Can you work these out from the model? Positions are in its coordinate system, mm. A direction names the side the tool comes from. Round coordinates to 2 decimals unless told otherwise and drop trailing zeros. Order: outer loops, then holes, each group sorted by start corner. A loop starts at its lowest first (then second) coordinate and runs counter-clockwise, first axis right, second up. Notation, with made-up numbers: (27.25, 24.5) -> (46.25, 24.5) arc R23 ccw to (46.25, 49.5) -> close; hole circle Ø2 at (-11.75, 75.5). An arc over 180 degrees is marked (long way). One line per item, written item: value.
```python
from build123d import *

# Parameters (mm, degrees)
ESQUISSE1_W      = 60
ESQUISSE1_H      = 33
ESQUISSE1_R      = 1.5
EXTRUSION1_DEPTH = 3
ESQUISSE2_W      = 7.634201779
ESQUISSE2_H      = 7.63420178
ESQUISSE2_W_2    = 5.337752956
ESQUISSE2_H_2    = 14.027301674
ESQUISSE2_W_3    = 5.224355128
ESQUISSE2_H_3    = 5.224355128
EXTRUSION2_DEPTH = 18
ESQUISSE3_R      = 3.279080348
EXTRUSION3_DEPTH = 12
ESQUISSE4_W      = 4
ESQUISSE4_H      = 19.646099489
EXTRUSION4_DEPTH = 23


with BuildPart() as part:
    # Esquisse1 → Extrusion1 (new body)
    with BuildSketch(Plane(origin=(0, 0, 0), x_dir=(1, 0, 0), z_dir=(0, 1, 0))):
        with Locations((30, 16.5)):
            Rectangle(ESQUISSE1_W, ESQUISSE1_H)
        with Locations((2.75, 29.5)):
            Circle(ESQUISSE1_R, mode=Mode.SUBTRACT)
        with Locations((57.25, 29.5)):
            Circle(ESQUISSE1_R, mode=Mode.SUBTRACT)
        with Locations((57.25, 3.5)):
            Circle(ESQUISSE1_R, mode=Mode.SUBTRACT)
        with Locations((2.75, 3.5)):
            Circle(ESQUISSE1_R, mode=Mode.SUBTRACT)
    extrude(amount=EXTRUSION1_DEPTH)

    # Esquisse2 → Extrusion2 (add)
    with BuildSketch(Plane(origin=(0, 3, 0), x_dir=(1, 0, 0), z_dir=(0, 1, 0))):
        with Locations((33.593446124, 26.205676479)):
            Rectangle(ESQUISSE2_W, ESQUISSE2_H)
        with Locations((51.457386868, 17.801055276)):
            Rectangle(ESQUISSE2_W_2, ESQUISSE2_H_2)
        with Locations((11.46939236, 25.577155504)):
            Rectangle(ESQUISSE2_W_3, ESQUISSE2_H_3)
        with Locations((22.552159567, 25.577155504)):
            Rectangle(ESQUISSE2_W_3, ESQUISSE2_H_3)
    extrude(amount=EXTRUSION2_DEPTH)

    # Esquisse3 → Extrusion3 (add)
    with BuildSketch(Plane(origin=(0, 3, 0), x_dir=(1, 0, 0), z_dir=(0, 1, 0))):
        with Locations((14, 8.756763264)):
            Circle(ESQUISSE3_R)
        with Locations((22, 8.756763264)):
            Circle(ESQUISSE3_R)
        with Locations((30, 8.756763264)):
            Circle(ESQUISSE3_R)
        with Locations((38, 8.756763264)):
            Circle(ESQUISSE3_R)
    extrude(amount=EXTRUSION3_DEPTH)

    # Esquisse4 → Extrusion4 (add)
    with BuildSketch(Plane(origin=(0, 3, 0), x_dir=(1, 0, 0), z_dir=(0, 1, 0))):
        with Locations((43.737455539, 15.895279312)):
            Rectangle(ESQUISSE4_W, ESQUISSE4_H)
    extrude(amount=EXTRUSION4_DEPTH)


solid = part.part
```
Q1. I want a section at B-B on z = -3.5. List the corners of the cut face in (x, y) for me, plus the area to 3 significant figures.
Answers below:
outline: (0, 0) -> (1.25, 0) -> (1.25, 3) -> (0, 3) -> close; (4.25, 0) -> (55.75, 0) -> (55.75, 3) -> (4.25, 3) -> close; (58.75, 0) -> (60, 0) -> (60, 3) -> (58.75, 3) -> close
area: 162 mm^2
Q2. I want a section at A-A on x = 2.75. List the corners of the cut face in (y, z) for me, plus the area to 3 significant figures.
Answers below:
outline: (0, -33) -> (3, -33) -> (3, -31) -> (0, -31) -> close; (0, -28) -> (3, -28) -> (3, -5) -> (0, -5) -> close; (0, -2) -> (3, -2) -> (3, 0) -> (0, 0) -> close
area: 81.0 mm^2
Q3. Please list where these lines run through material, in increasing order: line 1 along X through (y, z) = (12, -24.5); line 2 along Z through (x, y) = (57.25, 1.45); line 3 along X through (y, z) = (2.25, -29.5).
Answers below:
line 1: 8.86 to 14.08, 19.94 to 25.16, 29.78 to 37.41, 41.74 to 45.74, 48.79 to 54.13
line 2: -33 to -31, -28 to -5, -2 to 0
line 3: 0 to 1.25, 4.25 to 55.75, 58.75 to 60
Q4. We'd pull the mould along X, two halves only. Please class faces 1 (the face through (8.857, 12, -26)), 2 (the face through (51, 21, -18)), 3 (the face through (58.68, 1.48, -29.95)): released by +X, released by -X, zero draft, split by the parting line, or undercut.
Answers below:
face 1: released by -X
face 2: zero draft
face 3: undercut
Q5. I want a section at C-C on z = -27. List the corners of the cut face in (x, y) for me.
Answers below:
outline: (0, 0) -> (60, 0) -> (60, 3) -> (37.41, 3) -> (37.41, 21) -> (29.78, 21) -> (29.78, 3) -> (25.16, 3) -> (25.16, 21) -> (19.94, 21) -> (19.94, 3) -> (14.08, 3) -> (14.08, 21) -> (8.86, 21) -> (8.86, 3) -> (0, 3) -> close
Q6. Will these pins go through, and if not, where does the flat tip stop? pin 1 Ø3.5 at (x, z) = (12.5, -9) entering from +Y; pin 2 Ø2 at (x, y) = (44, 15.5) entering from +Z; pin 3 Ø4 at (x, y) = (16, 22.5) entering from -Z; pin 4 Ø5 at (y, z) = (22, -5.5) entering from +X.
Answers below:
pin 1: y = 15
pin 2: z = -6.07
pin 3: through
pin 4: x = 45.74
Q7. On a 3-axis mill with a long thin cutter (end or side, diameter ignored), from which of +Z, -Z, +X, -X, +Y, -Y can I reach the whole of each face in a straight line? I mean faces 4 (the face through (54.126, 12, -18)), 5 (the face through (45.737, 14, -16)), 6 (the face through (22, 15, -9)), 7 (the face through (34, 21, -26)). Say none if no direction works.
Answers below:
face 4: +Z, -Z, +X, +Y
face 5: +Z, -Z, +Y
face 6: +Z, -X, +Y
face 7: +Z, -Z, -X, +Y
Q8. I want a section at D-D on x = 38. List the corners of the cut face in (y, z) for me, plus the area to 3 significant figures.
Answers below:
outline: (0, -33) -> (3, -33) -> (3, -12.04) -> (15, -12.04) -> (15, -5.48) -> (3, -5.48) -> (3, 0) -> (0, 0) -> close
area: 178 mm^2
